Can you work these out from the model? Positions are in its coordinate system, mm. Give positions to 0.01 mm unless a question says otherwise; leave off trailing zeros. Loops run counter-clockwise (first coordinate to the right, second up) from the corner with the lowest first, then second, coordinate; pieces in that order, holes last. Notation, with made-up numbers: (42.5, 3.5) -> (80.5, 3.5) arc R18 ccw to (80.5, 9.5) -> close; hole circle Ø3 at (29, 72.5). An arc over 180 degrees is marked (long way). Use CSV: the item, a comma, the result in double quotes.
from build123d import *

# Parameters (mm, degrees)
SKETCH1_R           = 8
SKETCH1_R_2         = 2.05
BOSS_EXTRUDE1_DEPTH = 1.5875
FILLET1_R           = 1.5875


with BuildPart() as part:
    # Sketch1 → Boss-Extrude1 (new body)
    with BuildSketch(Plane.XY):
        with BuildLine():
            ThreePointArc((-165.1, 8.400260413), (-169.399739587, 11.575260413), (-174.625, 12.7))
            ThreePointArc((-174.625, 12.7), (-187.325, 0), (-174.625, -12.7))
            ThreePointArc((-174.625, -12.7), (-169.399739587, -11.575260413), (-165.1, -8.400260413))
            Line((-165.1, -8.400260413), (-165.1, 8.400260413))
        make_face()
        with Locations((-174.625, 0)):
            Circle(SKETCH1_R, mode=Mode.SUBTRACT)
        with BuildLine():
            Line((-165.1, 12.7), (-174.625, 12.7))
            ThreePointArc((-174.625, 12.7), (-169.399739587, 11.575260413), (-165.1, 8.400260413))
            Line((-165.1, 8.400260413), (-165.1, 12.7))
        make_face()
        with BuildLine():
            Line((-139.7, 12.7), (-165.1, 12.7))
            Line((-165.1, 12.7), (-165.1, 8.400260413))
            ThreePointArc((-165.1, 8.400260413), (-162.745237797, 4.490128061), (-161.925, 0))
            ThreePointArc((-161.925, 0), (-162.745237797, -4.490128061), (-165.1, -8.400260413))
            Line((-165.1, -8.400260413), (-165.1, -12.7))
            Line((-165.1, -12.7), (-139.7, -12.7))
            Line((-139.7, -12.7), (-139.7, 12.7))
        make_face()
        with Locations((-146.05, -6.35)):
            Circle(SKETCH1_R_2, mode=Mode.SUBTRACT)
        with Locations((-158.75, 6.35)):
            Circle(SKETCH1_R_2, mode=Mode.SUBTRACT)
        with BuildLine():
            ThreePointArc((-161.925, 0), (-162.745237797, 4.490128061), (-165.1, 8.400260413))
            Line((-165.1, 8.400260413), (-165.1, -8.400260413))
            ThreePointArc((-165.1, -8.400260413), (-162.745237797, -4.490128061), (-161.925, 0))
        make_face()
        with BuildLine():
            ThreePointArc((-165.1, -8.400260413), (-169.399739587, -11.575260413), (-174.625, -12.7))
            Line((-174.625, -12.7), (-165.1, -12.7))
            Line((-165.1, -12.7), (-165.1, -8.400260413))
        make_face()
    extrude(amount=BOSS_EXTRUDE1_DEPTH)

    # Fillet1
    fillet1_edges = [part.edges().sort_by_distance(p)[0] for p in [
        (-139.7, 12.7, 0.79375),
        (-139.7, -12.7, 0.79375),
    ]]
    fillet(fillet1_edges, radius=FILLET1_R)


solid = part.part
(1) Will this pin go through, and if not, where does the flat tip stop? pin 1 Ø3.5 at (x, y) = (-146.05, -6.35) entering from -Z.
Answer sheet:
pin 1,"passes through"
(2) If I drill on L1, parallel to Y at x = -158.75, z = 0.5; L2, parallel to Y at x = -146.05, z = 1.1; L3, parallel to X at y = -6, z = 1.2, over which ranges is the centre line in solid material (lowest first)? Write a range as from..to.
Answer sheet:
L1,"y = -12.7..4.3, 8.4..12.7"
L2,"y = -12.7..-8.4, -4.3..12.7"
L3,"x = -185.82..-179.92, -169.33..-148.07, -144.03..-139.7"
(3) We'd pull the mould along X, two halves only. Please class faces 1 (the face through (-140.18, 12.25, 0.8)), 2 (the face through (-147.677, -7.597, 0.783)), 3 (the face through (-187.32, 0.28, 0.78)): released by +X, released by -X, zero draft, split by the parting line, or undercut.
Answer sheet:
face 1,"released by +X"
face 2,"undercut"
face 3,"released by -X"
(4) If we section it at B-B, the plane y = 0: Write out the boundary of the cut face in (x, z) (1 decimal), then the cut area to 3 significant figures.
Answer sheet:
outline,"(-187.3, 0) -> (-182.6, 0) -> (-182.6, 1.6) -> (-187.3, 1.6) -> close; (-166.6, 0) -> (-139.7, 0) -> (-139.7, 1.6) -> (-166.6, 1.6) -> close"
area,"50.2 mm2"
(5) If we section it at A-A, the plane z = 1.15: Give the number of separate pieces and of enclosed holes in the cut face, then the cut area to 3 significant figures.
Answer sheet:
separate pieces,"1"
enclosed holes,"3"
area,"912 mm2"
(6) If we section it at C-C, the plane x = -158.75: Write out the boundary of the cut face in (y, z), then the cut area to 3 significant figures.
Answer sheet:
outline,"(-12.7, 0) -> (4.3, 0) -> (4.3, 1.59) -> (-12.7, 1.59) -> close; (8.4, 0) -> (12.7, 0) -> (12.7, 1.59) -> (8.4, 1.59) -> close"
area,"33.8 mm2"
(7) If we section it at D-D, the plane y = 6.35: Write out the boundary of the cut face in (x, z), then the cut area to 3 significant figures.
Answer sheet:
outline,"(-185.62, 0) -> (-179.49, 0) -> (-179.49, 1.59) -> (-185.62, 1.59) -> close; (-169.76, 0) -> (-160.8, 0) -> (-160.8, 1.59) -> (-169.76, 1.59) -> close; (-156.7, 0) -> (-139.7, 0) -> (-139.7, 1.59) -> (-156.7, 1.59) -> close"
area,"50.9 mm2"
